from build123d import *

# Parameters (mm, degrees)
SKETCH1_R                                    = 23
BOSS_EXTRUDE1_DEPTH                          = 17
SHELL1_T                                     = -2.6
SKETCH4_R                                    = 4.5
BOSS_EXTRUDE3_DEPTH                          = 5
SKETCH5_R                                    = 3.265
CUT_EXTRUDE2_DEPTH                           = 34.857938508
M1_6_TAPPED_HOLE1_D                          = 1.25
BOSS_EXTRUDE8_START                          = 5
SKETCH20_W                                   = 3
SKETCH20_H                                   = 3
SKETCH20_R                                   = 0.625
BOSS_EXTRUDE8_DEPTH                          = 5
SKETCH22_R                                   = 20.4
SKETCH22_R_2                                 = 17.6
BOSS_EXTRUDE10_DEPTH                         = 14.4
SKETCH24_R                                   = 2.25
BOSS_EXTRUDE11_DEPTH                         = 6.8
CSK_SLOT_FOR_M1_6_COUNTERSUNK_FLAT_H_2_COUNT = 2
CSK_SLOT_FOR_M1_6_COUNTERSUNK_FLAT_H_2_PITCH = 27.712812921
CSK_SLOT_FOR_M1_6_COUNTERSUNK_FLAT_H_3_COUNT = 2
CSK_SLOT_FOR_M1_6_COUNTERSUNK_FLAT_H_3_PITCH = 27.712812921


with BuildPart() as part:
    # Sketch1 → Boss-Extrude1 (new body)
    with BuildSketch(Plane(origin=(0, 0, 0), x_dir=(1, 0, 0), z_dir=(0, 1, 0))):
        with Locations(Location((0, 0, 0), (0, 0, 270))):
            Circle(SKETCH1_R)
    extrude(amount=BOSS_EXTRUDE1_DEPTH)

    # Shell1
    shell1_openings = [part.faces().sort_by_distance(p)[0] for p in [
        (0, 17, 0),
    ]]
    offset(amount=SHELL1_T, openings=shell1_openings, kind=Kind.INTERSECTION)

    # Sketch4 → Boss-Extrude3 (add)
    with BuildSketch(Plane(origin=(0, 2.6, 0), x_dir=(1, 0, 0), z_dir=(0, 1, 0))):
        with Locations(Location((0, 0, 0), (0, 0, 270))):
            Circle(SKETCH4_R)
    extrude(amount=BOSS_EXTRUDE3_DEPTH)

    # Sketch5 → Cut-Extrude2 (cut, through all)
    with BuildSketch(Plane(origin=(0, 7.6, 0), x_dir=(1, 0, 0), z_dir=(0, 1, 0))):
        with Locations(Location((0, 0, 0), (0, 0, 270))):
            Circle(SKETCH5_R)
    extrude(amount=-CUT_EXTRUDE2_DEPTH, mode=Mode.SUBTRACT)

    # M1.6 Tapped Hole1 (through all)
    with Locations(Plane(origin=(0, 0, 0), x_dir=(-1, 0, 0), z_dir=(0, -1, 0))):
        with Locations((0, 6.497951731), (0, -6.497951731)):
            Hole(M1_6_TAPPED_HOLE1_D / 2)

    # Sketch20 → Boss-Extrude8 (add)
    # profile 1 of 2: a face of its own
    with BuildSketch(Plane(origin=(0, 2.6, 0), x_dir=(1, 0, 0), z_dir=(0, 1, 0)).offset(BOSS_EXTRUDE8_START)):
        with Locations((0, -6.497951731)):
            Rectangle(SKETCH20_W, SKETCH20_H)
        with Locations(Location((0, -6.497951731, 0), (0, 0, 90))):
            Circle(SKETCH20_R, mode=Mode.SUBTRACT)
    # profile 2 of 2: a face of its own
    with BuildSketch(Plane(origin=(0, 2.6, 0), x_dir=(1, 0, 0), z_dir=(0, 1, 0)).offset(BOSS_EXTRUDE8_START)):
        with Locations((0, 6.497951731)):
            Rectangle(SKETCH20_W, SKETCH20_H)
        with Locations(Location((0, 6.497951731, 0), (0, 0, 90))):
            Circle(SKETCH20_R, mode=Mode.SUBTRACT)
    extrude(amount=-BOSS_EXTRUDE8_DEPTH)

    # Sketch22 → Boss-Extrude10 (add)
    with BuildSketch(Plane(origin=(0, 2.6, 0), x_dir=(1, 0, 0), z_dir=(0, 1, 0))):
        Circle(SKETCH22_R)
        with Locations(Location((0, 0, 0), (0, 0, 270))):
            Circle(SKETCH22_R_2, mode=Mode.SUBTRACT)
    extrude(amount=BOSS_EXTRUDE10_DEPTH)

    # Sketch24 → Boss-Extrude11 (add)
    with BuildSketch(Plane(origin=(0, 2.6, 0), x_dir=(1, 0, 0), z_dir=(0, 1, 0))):
        with Locations((-8, 13.856406461)):
            Circle(SKETCH24_R)
        with Locations((16, 0)):
            Circle(SKETCH24_R)
        with Locations((-8, -13.856406461)):
            Circle(SKETCH24_R)
    extrude(amount=BOSS_EXTRUDE11_DEPTH)

    # Sketch26 → CSK SLOT for M1.6 Countersunk Flat Head (revolve, cut)
    with BuildSketch(Plane(origin=(-8, 0, 13.856406461), x_dir=(0, 0, -1), z_dir=(1, 0, 0))):
        Polygon((0, 0), (0, 17), (0.9, 17), (0.9, 8.4), (1.8, 7.5), (1.8, 0), align=None)
    csk_slot_for_m1_6_countersunk_flat_head = revolve(axis=Axis((-8, -6.35, 13.856406461), (0, 1, 0)), mode=Mode.SUBTRACT)

    # CSK SLOT for M1.6 Countersunk Flat H 2: CSK SLOT for M1.6 Countersunk Flat Head ×2
    with Locations(*[(0, 0, -i * CSK_SLOT_FOR_M1_6_COUNTERSUNK_FLAT_H_2_PITCH) for i in range(1, CSK_SLOT_FOR_M1_6_COUNTERSUNK_FLAT_H_2_COUNT)]):
        add(csk_slot_for_m1_6_countersunk_flat_head, mode=Mode.SUBTRACT)

    # CSK SLOT for M1.6 Countersunk Flat H 3: CSK SLOT for M1.6 Countersunk Flat Head ×2
    with Locations(*[Vector(0.8660254037844364, 0, -0.5000000000000041) * (i * CSK_SLOT_FOR_M1_6_COUNTERSUNK_FLAT_H_3_PITCH) for i in range(1, CSK_SLOT_FOR_M1_6_COUNTERSUNK_FLAT_H_3_COUNT)]):
        add(csk_slot_for_m1_6_countersunk_flat_head, mode=Mode.SUBTRACT)


solid = part.part
Design review of the part built by this model. Coordinates are the model's own, in mm. A direction names the side the tool comes from. Round coordinates to 2 decimals unless told otherwise and drop trailing zeros. Write each loop counter-clockwise with the first axis right and the second up, starting at its lowest first coordinate (ties: lowest second). Pieces come first, ordered by that corner, then holes. Notation, with made-up numbers: (71, 65) - (78, 65) arc R22 cw to (78, 85) - close; hole circle Ø7 at (26.25, 16). An arc over 180 degrees is marked (long way). Return JSON: item names as keys, results as strings. Group by question number.
Item 1: We need section A-A on z = 0. Write out the cut boundary in (x, y) (3 decimals).
Item 2: The part is to be moulded in two halves that separate along Z. For faces 4 (the face through (19.394, 8.381, 12.365)), 5 (the face through (0, 5, -4.998)), 6 (the face through (-5, 0, 0)), 7 (the face through (0, 5, -7.998)), say which applies: pulls with the +Z half, pulls with the -Z half, needs draft (parallel to the pull), parting line crosses it, or undercut.
Item 3: Machinability: for faces 1 (the face through (-6.403, 3.698, -14.687)), 2 (the face through (-1.5, 5, 7)), 3 (the face through (0.491, 3.853, 6.884)), which of the approach directions +Z, -Z, +X, -X, +Y, -Y give a long, thin tool a straight path to every point of the face, cutting with its end or side? Answer none if there is none.
Item 4: For probe 1 along X at (y, z) = (9.25, 0); probe 2 along X at (y, z) = (7.25, 4); probe 3 along X at (y, z) = (7.5, 1), list the stretches that pass through material, from the lowest coordinate up. Write a range as [from, to].
Item 5: Insertion check: P1, Ø3, axis at x = -8, z = 13.86, coming from the +Y side; P2, Ø2, axis at y = 10, z = 16.5, coming from the -X side; P3, Ø3.5, axis at y = 4.5, z = -6.5, coming from the -X side. Each pin has a flat end and moves straight along its axis. Give the tip position at first contact, or say it passes through.
Item 6: We need section C-C on x = 16. Write out the cut boundary in (y, z), and give its area (3 significant figures).
Item 7: We need section B-B on y = 5.5. Give the number of separate pieces and of enclosed holes in the cut face, and give its area (3 significant figures).
Item 8: We need section D-D on y = 15.5. Write out the cut boundary in (x, z), and give its area (3 significant figures).
Model answer:
{
 "1": {"outline": "(-23, 0) - (-3.265, 0) - (-3.265, 7.6) - (-4.5, 7.6) - (-4.5, 2.6) - (-17.6, 2.6) - (-17.6, 17) - (-23, 17) - close; (3.265, 0) - (14.2, 0) - (14.2, 7.5) - (15.1, 8.4) - (15.1, 9.4) - (13.75, 9.4) - (13.75, 2.6) - (4.5, 2.6) - (4.5, 7.6) - (3.265, 7.6) - close; (16.9, 8.4) - (17.8, 7.5) - (17.8, 0) - (23, 0) - (23, 17) - (17.6, 17) - (17.6, 9.4) - (16.9, 9.4) - close"},
 "2": {"face 4": "parting line crosses it", "face 5": "undercut", "face 6": "needs draft", "face 7": "undercut"},
 "3": {"face 1": "-Y", "face 2": "+Y", "face 3": "+Y, -Y"},
 "4": {"probe 1": "x = [-23, -17.6], [13.75, 15.1], [16.9, 23]", "probe 2": "x = [-22.65, -17.14], [-2.06, 2.06], [17.14, 22.65]", "probe 3": "x = [-22.98, -17.57], [-4.39, -3.11], [3.11, 4.39], [13.98, 14.5], [17.5, 22.98]"},
 "5": {"P1": "stops at y = 9.4", "P2": "stops at x = -16.99", "P3": "stops at x = -22.5"},
 "6": {"outline": "(0, -16.52) - (17, -16.52) - (17, -7.33) - (2.6, -7.33) - (2.6, -2.25) - (9.4, -2.25) - (9.4, -0.9) - (8.4, -0.9) - (7.5, -1.8) - (0, -1.8) - close; (0, 1.8) - (7.5, 1.8) - (8.4, 0.9) - (9.4, 0.9) - (9.4, 2.25) - (2.6, 2.25) - (2.6, 7.33) - (17, 7.33) - (17, 16.52) - (0, 16.52) - close", "area": "350 mm²"},
 "7": {"separate pieces": "4", "enclosed holes": "7", "area": "747 mm²"},
 "8": {"outline": "circle Ø46 at (0, 0); hole circle Ø35.2 at (0, 0)", "area": "689 mm²"}
}
